Can you work these out from the model? Positions are in its coordinate system, mm. Face numbers are marked on the shaded views. A direction names the side the tool comes from. Round coordinates to 2 decimals unless told otherwise and drop trailing zeros. Order: outer loops, then holes, each group sorted by start corner. A loop starts at its lowest first (then second) coordinate and runs counter-clockwise, first axis right, second up. Notation, with made-up numbers: M -33.5,0.25 L 16.5,0.25 A13 ccw 16.5,17.25 Z; hole C 12,27.5 d3. An arc over 180 degrees is marked long. One line per question, with ' | ' between items.
```python
from build123d import *

# Parameters (mm, degrees)
SKETCH1_W           = 109
SKETCH1_H           = 59
SKETCH1_W_2         = 89
SKETCH1_H_2         = 39
BOSS_EXTRUDE1_DEPTH = 10
SKETCH2_W           = 109
SKETCH2_H           = 59
BOSS_EXTRUDE2_DEPTH = 10
SKETCH3_R           = 10.093684064
BOSS_EXTRUDE3_DEPTH = 10


with BuildPart() as part:
    # Sketch1 → Boss-Extrude1 (new body)
    with BuildSketch(Plane.XY):
        with Locations((54.5, -29.5)):
            Rectangle(SKETCH1_W, SKETCH1_H)
        with Locations((54.5, -29.5)):
            Rectangle(SKETCH1_W_2, SKETCH1_H_2, mode=Mode.SUBTRACT)
    extrude(amount=BOSS_EXTRUDE1_DEPTH)

    # Sketch2 → Boss-Extrude2 (add)
    with BuildSketch(Plane(origin=(0, 0, 0), x_dir=(-1, 0, 0), z_dir=(0, 0, -1))):
        with Locations((-54.5, -29.5)):
            Rectangle(SKETCH2_W, SKETCH2_H)
    extrude(amount=BOSS_EXTRUDE2_DEPTH)

    # Sketch3 → Boss-Extrude3 (add)
    with BuildSketch(Plane(origin=(0, 0, -10), x_dir=(-1, 0, 0), z_dir=(0, 0, -1))):
        with Locations((-54.5, -29.5)):
            Circle(SKETCH3_R)
    extrude(amount=BOSS_EXTRUDE3_DEPTH)


solid = part.part
```
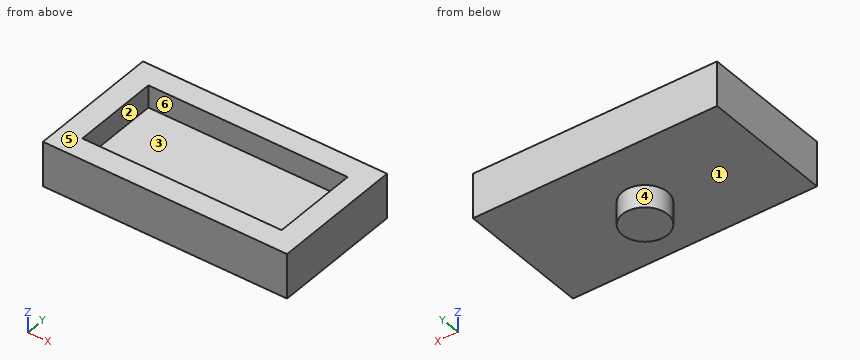
(1) Will these pins go through, and if not, where does the flat tip stop? pin 1 Ø1 at (y, z) = (-20, -14.5) entering from +X; pin 2 Ø6 at (x, y) = (31.5, -7.5) entering from -Z; pin 3 Ø11.5 at (x, y) = (70.5, -33) entering from +Z.
Final values:
pin 1: x = 59.07 | pin 2: z = -10 | pin 3: z = 0
(2) If we section it at D-D on z = -16.5: Please give me the cut outline in (x, y), plus the area to 3 significant figures.
Final values:
outline: C 54.5,-29.5 d20.19 | area: 320 mm^2
(3) On a 3-axis mill with a long thin cutter (end or side, diameter ignored), from which of +Z, -Z, +X, -X, +Y, -Y can I reach the whole of each face in a straight line? I mean the marked faces 5 and 6. Say none if no direction works.
Final values:
face 5: +Z, +X, -X, +Y, -Y | face 6: +Z
(4) If we section it at B-B on x = 68: Please give me the cut outline in (y, z).
Final values:
outline: M -59,-10 L 0,-10 L 0,10 L -10,10 L -10,0 L -49,0 L -49,10 L -59,10 Z
(5) Thinking about a two-plate mould opening in X: for the marked faces 1, 2, 3 and 4, which applies, released by +X, released by -X, zero draft, split by the parting line, or undercut?
Final values:
face 1: zero draft | face 2: undercut | face 3: undercut | face 4: split by the parting line
(6) If we section it at A-A on z = 6.5: Please give me the cut outline in (x, y), plus the area to 3 significant figures.
Final values:
outline: M 0,-59 L 109,-59 L 109,0 L 0,0 Z; hole M 10,-49 L 99,-49 L 99,-10 L 10,-10 Z | area: 2,960 mm^2
(7) Please list where these lines run through material, in increasing order: probe 1 along Y at (x, z) = (21.5, 5.75); probe 2 along X at (y, z) = (-32.5, 4.75); probe 3 along Z at (x, y) = (8.5, -47). Write a range as [from, to].
Final values:
probe 1: [-59, -49], [-10, 0] | probe 2: [0, 10], [99, 109] | probe 3: [-10, 10]
(8) If we section it at C-C on y = -29.5: Please give me the cut outline in (x, z), plus the area to 3 significant figures.
Final values:
outline: M 0,-10 L 44.41,-10 L 44.41,-20 L 64.59,-20 L 64.59,-10 L 109,-10 L 109,10 L 99,10 L 99,0 L 10,0 L 10,10 L 0,10 Z | area: 1,490 mm^2
